Autodesk Inventor part; units mm, degrees
ref_plane "YZ Plane" through (0, 0, 0) normal (1, 0, 0) x (0, 1, 0)
ref_plane "XZ Plane" through (0, 0, 0) normal (0, 1, 0) x (-1, 0, 0)
ref_plane "XY Plane" through (0, 0, 0) normal (0, 0, 1) x (1, 0, 0)
sketch "Sketch1" plane through (0, 0, 0) normal (0, 0, 1) x (1, 0, 0)
  line L0 (-27.45, -52.45) -> (27.45, -52.45) construction
  line L1 (52.45, -27.45) -> (52.45, 27.45) construction
  line L2 (27.45, 52.45) -> (-27.45, 52.45) construction
  line L3 (-52.45, 27.45) -> (-52.45, -27.45) construction
  line L4 (-52.45, -52.45) -> (52.45, 52.45) construction
  line L5 (52.45, -52.45) -> (-52.45, 52.45) construction
  arc A0 (-27.45, 52.45) -> (-52.45, 27.45) centre (-27.45, 27.45) ccw construction
  arc A1 (-52.45, -27.45) -> (-27.45, -52.45) centre (-27.45, -27.45) ccw construction
  arc A2 (27.45, -52.45) -> (52.45, -27.45) centre (27.45, -27.45) ccw construction
  arc A3 (52.45, 27.45) -> (27.45, 52.45) centre (27.45, 27.45) ccw construction
  line L6 (47.45, 27.45) -> (47.45, -27.45)
  arc A4 (27.45, -47.45) -> (47.45, -27.45) centre (27.45, -27.45) ccw
  line L7 (27.45, -47.45) -> (-27.45, -47.45)
  arc A5 (-47.45, -27.45) -> (-27.45, -47.45) centre (-27.45, -27.45) ccw
  line L8 (-47.45, -27.45) -> (-47.45, 27.45)
  arc A6 (-27.45, 47.45) -> (-47.45, 27.45) centre (-27.45, 27.45) ccw
  line L9 (-27.45, 47.45) -> (27.45, 47.45)
  arc A7 (47.45, 27.45) -> (27.45, 47.45) centre (27.45, 27.45) ccw
  line L10 (-35, 35) -> (35, 35) construction
  line L11 (35, 35) -> (35, -35) construction
  line L12 (35, -35) -> (-35, -35) construction
  line L13 (-35, -35) -> (-35, 35) construction
  line L14 (-35, 35) -> (35, -35) construction
  line L15 (35, 35) -> (-35, -35) construction
  circle A8 centre (35, 35) radius 2
  circle A9 centre (35, -35) radius 2
  circle A10 centre (-35, -35) radius 2
  circle A11 centre (-35, 35) radius 2
  point P0 (0, 0)
  dimension "d0" = 104.9
  dimension "d1" = 104.9
  dimension "d2" = 25
  dimension "d6" = 5
  dimension "d12" = 70
  dimension "d13" = 4
extrude "Extrusion1" add sketch "Sketch1" along normal blind 5
sketch "Sketch2" plane through (0, 0, 5) normal (0, 0, 1) x (1, 0, 0)
  line L0 (-30, 30) -> (30, 30)
  line L1 (30, 30) -> (30, -30)
  line L2 (30, -30) -> (-30, -30)
  line L3 (-30, 30) -> (30, -30) construction
  line L4 (30, 30) -> (-30, -30) construction
  line L5 (-64.9, 2) -> (-30, 2)
  line L6 (-30, -2) -> (-64.9, -2)
  line L7 (-64.9, -2) -> (-64.9, 2)
  line L8 (-47.45, 27.45) -> (-47.45, -27.45)
  line L9 (-64.9, 2) -> (-30, -2) construction
  line L10 (-30, 2) -> (-64.9, -2) construction
  line L11 (-30, -30) -> (-30, -2)
  line L12 (-30, 2) -> (-30, 30)
  point P0 (0, 0)
  point P1 (-47.45, 0)
  dimension "d7" = 4
  dimension "d8" = 60
  dimension "d9" = 60
extrude "Extrusion2" cut sketch "Sketch2" against normal blind 10
fillet "Fillet1" radius 5 4 edges at (30, 30, 2.5) (-30, 30, 2.5) (30, -30, 2.5) (-30, -30, 2.5)
equation "\"d1\" = d0"
equation "\"d9\" = d8"
properties part number "NewFront_H"
Geometry: final body of the model. Coordinates: model frame, mm. A direction names the side the tool comes from. Round coordinates to 2 decimals unless told otherwise and drop trailing zeros. Loops run counter-clockwise (first coordinate to the right, second up) from the corner with the lowest first, then second, coordinate; pieces in that order, holes last. Notation, with made-up numbers: M -0.75,25.5 L 42.25,25.5 A16 cw 42.25,56.5 Z; hole C -3,3.25 d9. An arc over 180 degrees is marked long. One line per question, with ' | ' between items.
(1) Material intervals for line 1 along Y through (x, z) = (6.5, 3.95); line 2 along Y through (x, z) = (-35, 1.2); line 3 along Y through (x, z) = (35, 1.15), sorted ascending. Write a range as from..to.
Check result:
line 1: y = -47.45..-30, 30..47.45 | line 2: y = -45.97..-37, -33..-2, 2..33, 37..45.97 | line 3: y = -45.97..-37, -33..33, 37..45.97
(2) Pull-direction query (Y, two-part tool) for faces 4 (the cylindrical face through (41.747, -41.436, 2.465)), 5 (the cylindrical face through (41.436, 41.747, 2.465)), 6 (the flat face through (30, 0, 3)); classes: +Y half, -Y half, draft (parallel to the pull), parting line (faces both ways), or undercut.
Check result:
face 4: -Y half | face 5: +Y half | face 6: undercut
(3) Contact query for a flat-ended pin moving along its axis: P1, Ø1.5, axis at x = -39, z = 3, coming from the -Y side. Output: stop coordinate, or through.
Check result:
P1: stops at y = -44.28
(4) Cut plane D-D on x = -35. Return the cut outline in (y, z).
Check result:
outline: M -45.97,0 L -37,0 L -37,5 L -45.97,5 Z; M -33,0 L -2,0 L -2,5 L -33,5 Z; M 2,0 L 33,0 L 33,5 L 2,5 Z; M 37,0 L 45.97,0 L 45.97,5 L 37,5 Z
(5) Cut plane B-B on x = -4.5. Return the cut outline in (y, z).
Check result:
outline: M -47.45,0 L -30,0 L -30,5 L -47.45,5 Z; M 30,0 L 47.45,0 L 47.45,5 L 30,5 Z
(6) Access query for faces 1 (the flat face through (-47.45, -15, 2)), 2 (the flat face through (0, -30, 3)), 3 (the flat face through (-39, 2, 3)). Directions: +Z, -Z, +X, -X, +Y, -Y. A direction counts if a zero-diameter tool reaches every point of the face in a straight line with its end or side. Return the directions, or none.
Check result:
face 1: +Z, -Z, -X, +Y, -Y | face 2: +Z, -Z | face 3: +Z, -Z, -X
(7) Cut plane A-A on z = 2.6. Return the cut outline in (x, y).
Check result:
outline: M -47.45,-27.45 A20 ccw -27.45,-47.45 L 27.45,-47.45 A20 ccw 47.45,-27.45 L 47.45,27.45 A20 ccw 27.45,47.45 L -27.45,47.45 A20 ccw -47.45,27.45 L -47.45,2 L -30,2 L -30,25 A5 cw -25,30 L 25,30 A5 cw 30,25 L 30,-25 A5 cw 25,-30 L -25,-30 A5 cw -30,-25 L -30,-2 L -47.45,-2 Z; hole C -35,-35 d4; hole C -35,35 d4; hole C 35,-35 d4; hole C 35,35 d4
